from build123d import *

# Parameters (mm, degrees)
SKETCH1_R           = 4
BOSS_EXTRUDE1_DEPTH = 325
CUT_EXTRUDE1_DEPTH  = 7.5
SKETCH3_R           = 4
SKETCH3_R_2         = 3.5
CUT_EXTRUDE2_DEPTH  = 1


with BuildPart() as part:
    # Sketch1 → Boss-Extrude1 (new body)
    with BuildSketch(Plane.XY):
        Circle(SKETCH1_R)
    extrude(amount=BOSS_EXTRUDE1_DEPTH)

    # Sketch2 → Cut-Extrude1 (cut)
    with BuildSketch(Plane.XY.offset(325)):
        with BuildLine():
            Line((3.122498999, 2.5), (-3.122498999, 2.5))
            ThreePointArc((-3.122498999, 2.5), (0, 4), (3.122498999, 2.5))
        make_face()
    extrude(amount=-CUT_EXTRUDE1_DEPTH, mode=Mode.SUBTRACT)

    # Sketch3 → Cut-Extrude2 (cut)
    with BuildSketch(Plane.XY.offset(323.75)):
        Circle(SKETCH3_R)
        Circle(SKETCH3_R_2, mode=Mode.SUBTRACT)
    extrude(amount=-CUT_EXTRUDE2_DEPTH, mode=Mode.SUBTRACT)


solid = part.part
Here's how the part is built. I have some questions about the finished solid (model axes, mm). A direction names the side the tool comes from. Coordinates: 2 decimals unless noted, no trailing zeros. Order: outer loops, then holes, each group sorted by start corner. A loop starts at its lowest first (then second) coordinate and runs counter-clockwise, first axis right, second up. Notation, with made-up numbers: M 62.5,58.25 L 86.5,58.25 A22 ccw 86.5,96.25 Z; hole C -0.75,-14 d7. An arc over 180 degrees is marked long. Answer as CSV lines item,"result".
Item 1: For pin 1 (1.2 mm diameter, centred on x = -0.5, y = 3, fed in from +Z); pin 2 (2 mm diameter, centred on y = -2.5, z = 229.5, fed in from -X); pin 3 (1 mm diameter, centred on x = 2, z = 209.5, fed in from +Y); pin 4 (3 mm diameter, centred on x = 1.5, z = 322.5, fed in from +Y), each with a flat end and sliding along its axis, tell me the tip position at first contact or that it passes through.
Results found:
pin 1,"z = 325"
pin 2,"x = -3.71"
pin 3,"y = 3.71"
pin 4,"y = 2.5"
Item 2: If I drill on line 1 (Z direction, x = 3.5, y = -1.75); line 2 (X direction, y = 0.25, z = 187.5); line 3 (Y direction, x = -2, z = 228.5), over which ranges is the centre line in solid material (lowest first)?
Results found:
line 1,"0 to 322.75, 323.75 to 325"
line 2,"-3.99 to 3.99"
line 3,"-3.46 to 3.46"
Item 3: Imagine slicing it at A-A on y = -2.25. Write out the boundary of the cut face in (x, z), plus the area to 3 significant figures.
Results found:
outline,"M -3.31,0 L 3.31,0 L 3.31,322.75 L 2.68,322.75 L 2.68,323.75 L 3.31,323.75 L 3.31,325 L -3.31,325 L -3.31,323.75 L -2.68,323.75 L -2.68,322.75 L -3.31,322.75 Z"
area,"2,150 mm2"
Item 4: On a 3-axis mill with a long thin cutter (end or side, diameter ignored), from which of +Z, -Z, +X, -X, +Y, -Y can I reach the whole of each face in a straight line? I mean faces 1 (the face through (0, -4, 324)), 2 (the face through (0, 2.5, 321)), 3 (the face through (-0.1, -3.5, 323.3)). Say none if no direction works.
Results found:
face 1,"+Z, -Z"
face 2,"+Z, +X, -X, +Y"
face 3,"none"
Item 5: Imagine slicing it at B-B on z = 77.5. Write out the boundary of the cut face in (x, y), plus the area to 3 significant figures.
Results found:
outline,"C 0,0 d8"
area,"50.3 mm2"
Item 6: We'd pull the mould along Z, two halves only. Please class faces 4 (the face through (-0.867, -3.905, 159.116)), 5 (the face through (0, 0, 0)), 6 (the face through (-0.61, -3.62, 323.75)): +Z half, -Z half, draft (parallel to the pull), parting line (faces both ways), or undercut.
Results found:
face 4,"draft"
face 5,"-Z half"
face 6,"undercut"
